```python
from build123d import *

# Parameters (mm, degrees)
SKETCH1_W           = 15
SKETCH1_H           = 40
SKETCH1_R           = 3.2
BOSS_EXTRUDE1_DEPTH = 2.5


with BuildPart() as part:
    # Sketch1 → Boss-Extrude1 (new body, symmetric)
    with BuildSketch(Plane.XY):
        Rectangle(SKETCH1_W, SKETCH1_H)
        with Locations((0, 3.9595)):
            Circle(SKETCH1_R, mode=Mode.SUBTRACT)
    extrude(amount=BOSS_EXTRUDE1_DEPTH, both=True)


solid = part.part
```
CAD build for the part. Positions are in the model's coordinates, mm. Round coordinates to 2 decimals unless told otherwise and drop trailing zeros. Order: outer loops, then holes, each group sorted by start corner. A loop starts at its lowest first (then second) coordinate and runs counter-clockwise, first axis right, second up. Notation, with made-up numbers: (-34.5, 25.25) -> (-20.5, 25.25) arc R26 ccw to (-20.5, 42.25) -> close; hole circle Ø5 at (-11.5, 73.25). An arc over 180 degrees is marked (long way). One line per question, with ' | ' between items.
Q1. Probe probe 1 along Y at (x, z) = (0, -1.15); probe 2 along X at (y, z) = (5, -0.7); probe 3 along X at (y, z) = (6, 0.85). List the from-to ranges inside material, lowest first.
Completed:
probe 1: y = -20 to 0.76, 7.16 to 20 | probe 2: x = -7.5 to -3.03, 3.03 to 7.5 | probe 3: x = -7.5 to -2.47, 2.47 to 7.5
Q2. Slice it at A-A (x = 0). Write the cut outline in (y, z), then the cut area to 3 significant figures.
Completed:
outline: (-20, -2.5) -> (0.76, -2.5) -> (0.76, 2.5) -> (-20, 2.5) -> close; (7.16, -2.5) -> (20, -2.5) -> (20, 2.5) -> (7.16, 2.5) -> close | area: 168 mm^2
Q3. Slice it at B-B (y = 2). Write the cut outline in (x, z).
Completed:
outline: (-7.5, -2.5) -> (-2.53, -2.5) -> (-2.53, 2.5) -> (-7.5, 2.5) -> close; (2.53, -2.5) -> (7.5, -2.5) -> (7.5, 2.5) -> (2.53, 2.5) -> close
Q4. Two-plate mould, pull along Y, no slides. Class faces 1 (the flat face through (0, 20, 0)), 2 (the cylindrical face through (-0.694, 0.836, -0.035)), 3 (the flat face through (0, -20, 0)): released by +Y, released by -Y, zero draft, split by the parting line, or undercut.
Completed:
face 1: released by +Y | face 2: undercut | face 3: released by -Y
Q5. Slice it at C-C (z = 1.85). Write the cut outline in (x, y).
Completed:
outline: (-7.5, -20) -> (7.5, -20) -> (7.5, 20) -> (-7.5, 20) -> close; hole circle Ø6.4 at (0, 3.96)
